Verification items for the finished model (mm, model axes). A direction names the side the tool comes from. Coordinates: 2 decimals unless noted, no trailing zeros. Loops run counter-clockwise (first coordinate to the right, second up) from the corner with the lowest first, then second, coordinate; pieces in that order, holes last. Notation, with made-up numbers: (3, 19) - (35, 19) arc R18 ccw to (35, 36) - close; hole circle Ø7 at (57, 59.25). An arc over 180 degrees is marked (long way). One line per item, written item: value. Start each with the question number.
(1) Set-up check for faces 1 (the face through (11, 9, -0.5)), 2 (the face through (11, 6, -0.5)), 3 (the face through (13, 7.5, -0.5)): record each of +Z, -Z, +X, -X, +Y, -Y from which the full face is reachable in a straight line by a thin tool's end or side.
(2) Section check B-B (y = 13). Record the boundary of the cut face in (x, z), plus the area to 3 significant figures.
(3) Section check D-D (y = 7). Record the boundary of the cut face in (x, z), plus the area to 3 significant figures.
(4) Thickness scan on probe 1 along Y at (x, z) = (20, 0.75); probe 2 along Y at (x, z) = (3, 1.35); probe 3 along Z at (x, y) = (1.5, 27.25). Record the ranges inside material, lowest first. Write a range as [from, to].
(5) Section check A-A (x = 2). Record the boundary of the cut face in (y, z), plus the area to 3 significant figures.
(6) Gauge pin test, flat ends, axial feed: P1, Ø0.5, axis at x = 11, z = -0.5, coming from the -Y side; P2, Ø1.6, axis at x = 2, y = 2, coming from the -Z side; P3, Ø3, axis at x = 11.5, y = 21.5, coming from the -Z side; P4, Ø0.5, axis at y = 7.5, z = -0.5, coming from the +X side. Record the tip position at first contact, or that the pin passes through.
(7) Section check C-C (z = 1.2). Record the boundary of the cut face in (x, y), plus the area to 3 significant figures.
(8) Draft check along X on faces 4 (the face through (18.7, 1.94, 0.74)), 5 (the face through (22, 14, 1)), 6 (the face through (11, 8, -1)). Enter one of: +X half, -X half, draft (parallel to the pull), parting line (faces both ways), or undercut.
Autodesk Inventor part; units mm, degrees
ref_plane "YZ Plane" through (0, 0, 0) normal (1, 0, 0) x (0, 1, 0)
ref_plane "XZ Plane" through (0, 0, 0) normal (0, 1, 0) x (-1, 0, 0)
ref_plane "XY Plane" through (0, 0, 0) normal (0, 0, 1) x (1, 0, 0)
sketch "Sketch1" plane through (0, 0, 0) normal (0, 0, 1) x (1, 0, 0)
  line L0 (0, 0) -> (0, 28)
  line L1 (0, 28) -> (22, 28)
  line L2 (22, 28) -> (22, 0)
  line L3 (22, 0) -> (0, 0)
  circle A0 centre (2, 13) radius 1.3
  circle A1 centre (20, 13) radius 1.3
  circle A2 centre (2, 2) radius 1.3
  circle A3 centre (20, 2) radius 1.3
  line L4 (11, 28) -> (11, 0) construction
  line L5 (2, 13) -> (20, 13) construction
  line L6 (2, 2) -> (20, 2) construction
  line L7 (9, 9) -> (13, 9)
  line L8 (13, 9) -> (13, 6)
  line L9 (13, 6) -> (9, 6)
  line L10 (9, 6) -> (9, 9)
  line L11 (2, 13) -> (2, 2)
  line L12 (9, 7.5) -> (13, 7.5) construction
  line L13 (11, 13) -> (11, 2) construction
  point P0 (11, 9)
  point P1 (11, 7.5)
  dimension "d0" = 28
  dimension "d1" = 22
  dimension "d2" = 2.6
  dimension "d5" = 18
  dimension "d8" = 11
  dimension "d11" = 2
  dimension "d14" = 4
  dimension "d15" = 3
extrude "Extrusion1" add sketch "Sketch1" along normal blind 1.5 contours L0 L1 L2 L3 | L7 L8 L9 L10
extrude "Extrusion2" add sketch "Sketch1" against normal blind 1 contours L7 L8 L9 L10
properties part number "Encoder"
Responses:
1. face 1: -Z, +X, -X, +Y
1. face 2: -Z, +X, -X, -Y
1. face 3: -Z, +X, +Y, -Y
2. outline: (0, 0) - (0.7, 0) - (0.7, 1.5) - (0, 1.5) - close; (3.3, 0) - (18.7, 0) - (18.7, 1.5) - (3.3, 1.5) - close; (21.3, 0) - (22, 0) - (22, 1.5) - (21.3, 1.5) - close
2. area: 25.2 mm²
3. outline: (0, 0) - (9, 0) - (9, -1) - (13, -1) - (13, 0) - (22, 0) - (22, 1.5) - (0, 1.5) - close
3. area: 37.0 mm²
4. probe 1: y = [0, 0.7], [3.3, 11.7], [14.3, 28]
4. probe 2: y = [0, 1.17], [2.83, 12.17], [13.83, 28]
4. probe 3: z = [0, 1.5]
5. outline: (0, 0) - (0.7, 0) - (0.7, 1.5) - (0, 1.5) - close; (3.3, 0) - (11.7, 0) - (11.7, 1.5) - (3.3, 1.5) - close; (14.3, 0) - (28, 0) - (28, 1.5) - (14.3, 1.5) - close
5. area: 34.2 mm²
6. P1: stops at y = 6
6. P2: passes through
6. P3: stops at z = 0
6. P4: stops at x = 13
7. outline: (0, 0) - (22, 0) - (22, 28) - (0, 28) - close; hole circle Ø2.6 at (2, 2); hole circle Ø2.6 at (2, 13); hole circle Ø2.6 at (20, 2); hole circle Ø2.6 at (20, 13)
7. area: 595 mm²
8. face 4: undercut
8. face 5: +X half
8. face 6: draft
